CAD build for the part. Positions are in the model's coordinates, mm. Face numbers are marked on the shaded views. Give positions to 0.01 mm unless a question says otherwise; leave off trailing zeros. Loops run counter-clockwise (first coordinate to the right, second up) from the corner with the lowest first, then second, coordinate; pieces in that order, holes last. Notation, with made-up numbers: M 35.25,-33.75 L 94.25,-33.75 A23 ccw 94.25,5.25 Z; hole C -7.75,42.5 d9. An arc over 180 degrees is marked long. Answer as CSV lines item,"result".
```python
from build123d import *

# Parameters (mm, degrees)
F1_ANGLE_BACK = 90
F1_ANGLE      = 180


with BuildPart() as f1:
    # F0 (on Front) → F1 (revolve)
    with BuildSketch(Plane.XZ, mode=Mode.PRIVATE) as f1_sk:
        Polygon((-95.25, -31.75), (-95.25, 0), (-101.6, 0), (-101.6, -38.1), (0, -38.1), (0, -31.75), align=None)
        with BuildLine():
            ThreePointArc((31.75, 0), (22.4506403027, -22.4506403027), (0, -31.75))
            Line((0, -31.75), (0, -38.1))
            ThreePointArc((0, -38.1), (26.9407683632, -26.9407683632), (38.1, 0))
            Line((38.1, 0), (31.75, 0))
        make_face()
    revolve(f1_sk.sketch.rotate(Axis((-50.8, 0, 0), (-1, 0, 0)), -F1_ANGLE_BACK), axis=Axis((-50.8, 0, 0), (-1, 0, 0)), revolution_arc=F1_ANGLE)


solid = f1.part
```
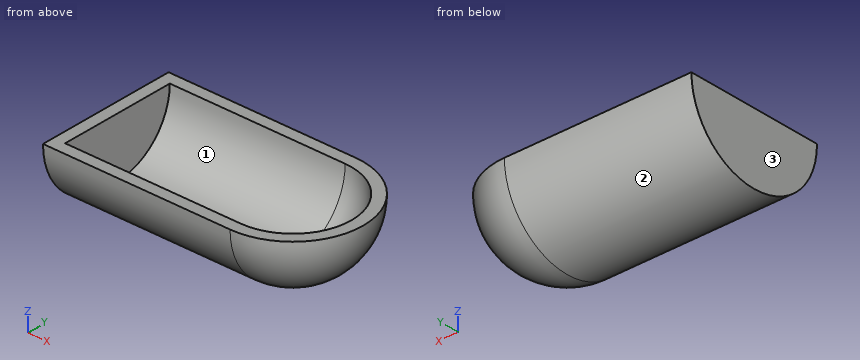
Q1. Cut at A-A (z = -18). Write the cut outline in (x, y).
Solution:
outline,"M -101.6,-33.58 L 0,-33.58 A33.58 ccw 0,33.58 L -101.6,33.58 Z; hole M -95.25,-26.15 L 0,-26.15 A26.15 ccw 0,26.15 L -95.25,26.15 Z"
Q2. Pin check, flat tips, straight feed: P1, Ø4, axis at x = -16.5, z = -33, coming from the -Y side; P2, Ø8, axis at x = -81.5, y = 14, coming from the +Z side; P3, Ø16, axis at y = -2, z = -23.5, coming from the +X side. Stop position of each tip, or through.
Solution:
P1,"stops at y = -22.15"
P2,"stops at z = -26.15"
P3,"stops at x = 34.77"
Q3. Cut at C-C (z = -11). Write the cut outline in (x, y), and give its area (3 significant figures).
Solution:
outline,"M -101.6,-36.48 L 0,-36.48 A36.48 ccw 0,36.48 L -101.6,36.48 Z; hole M -95.25,-29.78 L 0,-29.78 A29.78 ccw 0,29.78 L -95.25,29.78 Z"
area,"2,440 mm²"
Q4. Mould opens along X. For the marked faces 1, 2 and 3 say: released by +X, released by -X, zero draft, split by the parting line, or undercut.
Solution:
face 1,"undercut"
face 2,"zero draft"
face 3,"released by -X"
Q5. Cut at D-D (x = -20.5). Write the cut outline in (y, z).
Solution:
outline,"M -38.1,0 A38.1 ccw 38.1,0 L 31.75,0 A31.75 cw -31.75,0 Z"
Q6. Cut at B-B (y = 0). Write the cut outline in (x, z), and give its area (3 significant figures).
Solution:
outline,"M -101.6,-38.1 L 0,-38.1 A38.1 ccw 38.1,0 L 31.75,0 A31.75 cw 0,-31.75 L -95.25,-31.75 L -95.25,0 L -101.6,0 Z"
area,"1,200 mm²"
Q7. Wall check: line 1 (Y direction, x = -8, z = -8); line 2 (X direction, y = 18, z = -5.5); line 3 (X direction, y = -2, z = -14). Give the ranges that are in metal, low to high. Write a range as [from, to].
Solution:
line 1,"y = [-37.25, -30.73], [30.73, 37.25]"
line 2,"x = [-101.6, -95.25], [25.57, 33.13]"
line 3,"x = [-101.6, -95.25], [28.43, 35.38]"
